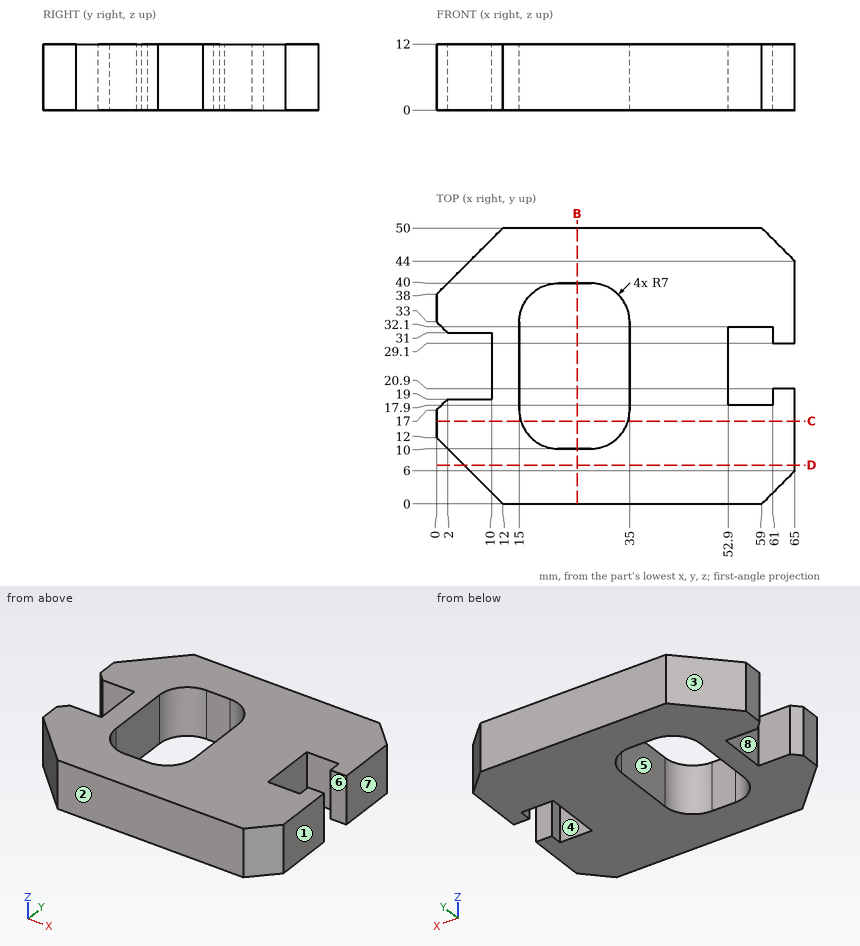
Answer from the drawing. Dimensions are ordinates in mm from the lowest x, y and z of the part. A direction names the side the tool comes from. Give positions to 0.01 mm unless a question says otherwise; leave off trailing zeros. Write each loop counter-clockwise with the first axis right and the second up, starting at its lowest first coordinate (ties: lowest second). Pieces come first, ordered by that corner, then holes. Notation, with made-up numbers: (-0.75, 27.5) - (17.25, 27.5) arc R32 cw to (17.25, 57.5) - close; hole circle Ø10 at (19.5, -34). An arc over 180 degrees is marked (long way). Answer in a Markdown table with one row per item. Add a question column.
Item 1: Find the intervals of material crossed by L1, parallel to X at y = 27, z = 11.5; L2, parallel to Y at x = 55.5, z = 4.5; L3, parallel to Y at x = 25, z = 9.25, in increasing order.
Item 2: Flat-ended cylindrical pins translate along their axes: P1, Ø6.5, axis at x = 7.5, z = 7, coming from the +Y side; P2, Ø6, axis at y = 23, z = 7.5, coming from the -X side; P3, Ø2.5, axis at y = 31, z = 7.5, coming from the -X side. Find the tip coordinate at first contact, or state that the pin passes through.
Item 3: Section B-B, the plane x = 25.5 is taken. Write down the section's boundary in (y, z).
Item 4: A tool of negligible diameter and unlimited length cuts with its end or side. For the marked faces 5, 6, 7 and 8, from which of +Z, -Z, +X, -X, +Y, -Y can it reach the whole face along a straight path? Write none if from no direction.
Item 5: Section D-D, the plane y = 7 is taken. Write down the section's boundary in (x, z), and give its area (3 significant figures).
Item 6: Section C-C, the plane y = 15 is taken. Write down the section's boundary in (x, z), and give its area (3 significant figures).
Item 7: Determine the mould class of the marked faces 1, 2, 3 and 4 for opening direction Y: pulls with the +Y half, pulls with the -Y half, needs draft (parallel to the pull), parting line crosses it, or undercut.
Recorded:
| question | item | result |
|---|---|---|
| 1 | L1 | x = 10 to 15, 35 to 52.9 |
| 1 | L2 | y = 0 to 17.9, 32.1 to 50 |
| 1 | L3 | y = 0 to 10, 40 to 50 |
| 2 | P1 | stops at y = 48.75 |
| 2 | P2 | stops at x = 10 |
| 2 | P3 | stops at x = 0.75 |
| 3 | outline | (0, 0) - (10, 0) - (10, 12) - (0, 12) - close; (40, 0) - (50, 0) - (50, 12) - (40, 12) - close |
| 4 | face 5 | +Z, -Z |
| 4 | face 6 | +Z, -Z, +X |
| 4 | face 7 | +Z, -Z, +X, +Y, -Y |
| 4 | face 8 | +Z, -Z, -X |
| 5 | outline | (5, 0) - (65, 0) - (65, 12) - (5, 12) - close |
| 5 | area | 720 mm2 |
| 6 | outline | (0, 0) - (15.29, 0) - (15.29, 12) - (0, 12) - close; (34.71, 0) - (65, 0) - (65, 12) - (34.71, 12) - close |
| 6 | area | 547 mm2 |
| 7 | face 1 | needs draft |
| 7 | face 2 | pulls with the -Y half |
| 7 | face 3 | pulls with the +Y half |
| 7 | face 4 | undercut |
